For this review, take the finished solid that the model builds, in its own axes (mm). A direction names the side the tool comes from. Round coordinates to 2 decimals unless told otherwise and drop trailing zeros. Loops run counter-clockwise (first coordinate to the right, second up) from the corner with the lowest first, then second, coordinate; pieces in that order, holes last. Notation, with made-up numbers: (34, 89) -> (44, 89) arc R25 cw to (44, 107) -> close; hole circle Ø4 at (26.25, 66). An arc over 180 degrees is marked (long way). One line per question, with ' | ' between items. Start each with the question number.
1. For pin 1 Ø3 at (y, z) = (-2.5, 2) entering from -X; pin 2 Ø1.5 at (x, z) = (4, 4.5) entering from +Y; pin 3 Ø12 at (x, y) = (-15.5, 22) entering from +Z; pin 4 Ø3.5 at (x, y) = (-3.5, 16) entering from +Z, all flat-tipped, find the tip position at first contact; note any pin that passes through.
2. Consider section C-C (y = 5.5). Write out the cut boundary in (x, z).
3. For faces 5 (the face through (5.9, -5.93, 2.96)), 6 (the face through (-11.75, 2, 3)), 7 (the face through (11.15, -11.43, 2.96)), 8 (the face through (-1, 10.5, 4)), list the 3-axis set-ups (+Z, -Z, +X, -X, +Y, -Y) from which the entire face can be reached by the end or side of a thin tool; tool diameter is ignored.
4. Consider section D-D (x = 9). Write out the cut boundary in (y, z).
5. Draft analysis for pull direction Y (two halves, no side actions). For faces 1 (the face through (-2, 8, 6)), 2 (the face through (-0.145, 23.161, 2.958)), 3 (the face through (-7.97, 18.69, 4.03)), 4 (the face through (7.75, -8.95, 2.96)), state which applies: pulls with the +Y half, pulls with the -Y half, needs draft (parallel to the pull), parting line crosses it, or undercut.
6. Wall thickness on line 1 along Y through (x, z) = (9, 1.7); line 2 along X through (y, z) = (2, 2.8); line 3 along Y through (x, z) = (-10, 2.7): over which ranges is each line inside the solid? List them lowest first.
7. Consider section A-A (z = 4.7). Count the separate pieces of the cut face and the enclosed holes in it, and give its area (3 significant figures).
8. Consider section B-B (y = -9). Write out the cut boundary in (x, z).
```python
from build123d import *

# Parameters (mm, degrees)
SKETCH_1_R          = 7.5
SKETCH_1_R_2        = 5
SKETCH_1_W          = 23.5
SKETCH_1_H          = 32
SKETCH_1_R_3        = 1.25
EXTRUDE_1_DEPTH     = 6
SKETCH_3_W          = 23.5
SKETCH_3_H          = 4
SKETCH_3_W_2        = 13
SKETCH_3_H_2        = 13
CUT_EXTRUDE_1_DEPTH = 7
CUT_EXTRUDE_2_DEPTH = 4
FILLET_2_R          = 2


with BuildPart() as part:
    # 草图1 → 凸台-拉伸1 (new body)
    # profile 1 of 3: a face of its own
    with BuildSketch(Plane.XY):
        with BuildLine():
            Line((-15.25, 16), (-11.75, 16))
            Line((-11.75, 16), (11.75, 16))
            Line((11.75, 16), (-11.381805158, 29.925501433))
            ThreePointArc((-11.381805158, 29.925501433), (-8.72077871, 27.190429425), (-7.75, 23.5))
            ThreePointArc((-7.75, 23.5), (-9.946699141, 18.196699141), (-15.25, 16))
        make_face()
    # profile 2 of 3: a face of its own
    with BuildSketch(Plane.XY):
        with Locations((-15.25, 23.5)):
            Circle(SKETCH_1_R)
        with Locations((-15.25, 23.5)):
            Circle(SKETCH_1_R_2, mode=Mode.SUBTRACT)
    # profile 3 of 3: a face of its own
    with BuildSketch(Plane.XY):
        Rectangle(SKETCH_1_W, SKETCH_1_H)
        with Locations((9, -9)):
            Circle(SKETCH_1_R_3, mode=Mode.SUBTRACT)
        with Locations((-9, -9)):
            Circle(SKETCH_1_R_3, mode=Mode.SUBTRACT)
        with Locations((-9, 9)):
            Circle(SKETCH_1_R_3, mode=Mode.SUBTRACT)
        with Locations((9, 9)):
            Circle(SKETCH_1_R_3, mode=Mode.SUBTRACT)
    extrude(amount=EXTRUDE_1_DEPTH)

    # 草图3 → 切除-拉伸1 (cut)
    with BuildSketch(Plane.XY.offset(6)):
        with Locations((0, -14)):
            Rectangle(SKETCH_3_W, SKETCH_3_H)
        Rectangle(SKETCH_3_W_2, SKETCH_3_H_2)
    extrude(amount=-CUT_EXTRUDE_1_DEPTH, mode=Mode.SUBTRACT)

    # 草图4 → 切除-拉伸2 (cut)
    with BuildSketch(Plane.XY.offset(6)):
        with BuildLine():
            Line((6.5, 15.658862876), (-6.525, 23.5))
            ThreePointArc((-6.525, 23.5), (-7.850272246, 18.877267672), (-11.423488063, 15.658862876))
            Line((-11.423488063, 15.658862876), (6.5, 15.658862876))
        make_face()
        Polygon((-6.5, 10.5), (6.5, 10.5), (6.5, 15.658862876), (-11.423488063, 15.658862876), align=None)
    extrude(amount=-CUT_EXTRUDE_2_DEPTH, mode=Mode.SUBTRACT)

    # 圆角2
    fillet_2_edges = [part.edges().sort_by_distance(p)[0] for p in [
        (11.75, 16, 3),
        (-11.75, 16, 3),
        (-11.75, -12, 3),
        (11.75, -12, 3),
        (6.5, 6.5, 3),
        (6.5, -6.5, 3),
        (-6.5, -6.5, 3),
        (-6.5, 6.5, 3),
        (-11.423488063, 15.658862876, 4),
        (-6.525, 23.5, 4),
        (6.5, 15.658862876, 4),
        (6.5, 10.5, 4),
        (-6.5, 10.5, 4),
    ]]
    fillet(fillet_2_edges, radius=FILLET_2_R)


solid = part.part
```
Answer block:
1) pin 1: stops at x = -11.75 | pin 2: stops at y = 21.12 | pin 3: stops at z = 6 | pin 4: stops at z = 2
2) outline: (-11.75, 0) -> (-6.23, 0) -> (-6.23, 6) -> (-11.75, 6) -> close; (6.23, 0) -> (11.75, 0) -> (11.75, 6) -> (6.23, 6) -> close
3) face 5: +Z, -Z | face 6: +Z, -Z, -X, -Y | face 7: +Z, -Z, +X, -Y | face 8: +Z
4) outline: (-12, 0) -> (-10.25, 0) -> (-10.25, 6) -> (-12, 6) -> close; (-7.75, 0) -> (7.75, 0) -> (7.75, 6) -> (-7.75, 6) -> close; (10.25, 0) -> (17.66, 0) -> (17.66, 6) -> (10.25, 6) -> close
5) face 1: needs draft | face 2: pulls with the +Y half | face 3: undercut | face 4: undercut
6) line 1: y = -12 to -10.25, -7.75 to 7.75, 10.25 to 17.66 | line 2: x = -11.75 to -6.5, 6.5 to 11.75 | line 3: y = -11.98 to -9.75, -8.25 to 8.25, 9.75 to 14.22, 16.4 to 29.09
7) separate pieces: 1 | enclosed holes: 7 | area: 562 mm2
8) outline: (-11.75, 0) -> (-10.25, 0) -> (-10.25, 6) -> (-11.75, 6) -> close; (-7.75, 0) -> (7.75, 0) -> (7.75, 6) -> (-7.75, 6) -> close; (10.25, 0) -> (11.75, 0) -> (11.75, 6) -> (10.25, 6) -> close
